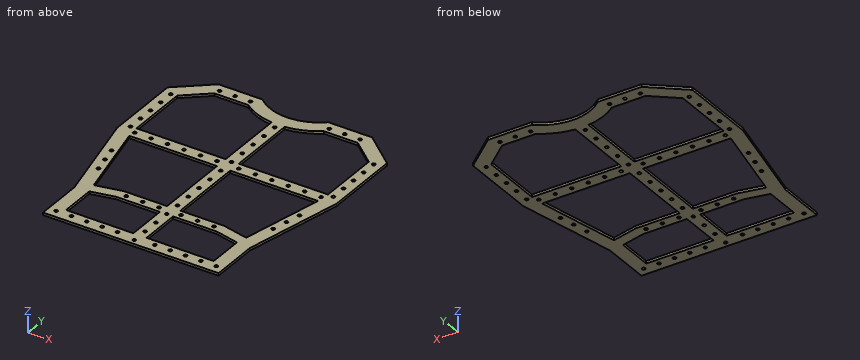
from build123d import *

# Parameters (mm, degrees)
BOSS_EXTRUDE1_DEPTH    = 2.286
SKETCH8_W              = 160
SKETCH8_H              = 1.5
CUT_EXTRUDE3_DEPTH     = 10
CUT_EXTRUDE4_DEPTH     = 3.286
BOSS_EXTRUDE2_DEPTH    = 2.286
F_3_0MM_DOWEL_HOLE4_D  = 3
F_3_0MM_DOWEL_HOLE5_D  = 3
F_3_0MM_DOWEL_HOLE6_D  = 3
F_3_0MM_DOWEL_HOLE7_D  = 3
F_3_0MM_DOWEL_HOLE8_D  = 3
F_3_0MM_DOWEL_HOLE9_D  = 3
F_3_0MM_DOWEL_HOLE10_D = 3


with BuildPart() as part:
    # Sketch1 → Boss-Extrude1 (new body)
    with BuildSketch(Plane.XY):
        with BuildLine():
            Line((-30, 6.458980338), (-70, 6.458980338))
            Line((-70, 6.458980338), (-100, -18.541019662))
            Line((-100, -18.541019662), (-100, -88.541019662))
            Line((-100, -88.541019662), (-80, -178.541019662))
            Line((-80, -178.541019662), (-80, -223.541019662))
            Line((-80, -223.541019662), (80, -223.541019662))
            Line((80, -223.541019662), (80, -178.541019662))
            Line((80, -178.541019662), (100, -88.541019662))
            Line((100, -88.541019662), (100, -18.541019662))
            Line((100, -18.541019662), (70, 6.458980338))
            Line((70, 6.458980338), (30, 6.458980338))
            ThreePointArc((30, 6.458980338), (0, -5), (-30, 6.458980338))
        make_face()
    extrude(amount=BOSS_EXTRUDE1_DEPTH)

    # Sketch8 → Cut-Extrude3 (cut)
    with BuildSketch(Plane.XY.offset(2.286)):
        with Locations((0, -222.791019662)):
            Rectangle(SKETCH8_W, SKETCH8_H)
    extrude(amount=-CUT_EXTRUDE3_DEPTH, mode=Mode.SUBTRACT)

    # Sketch15 → Cut-Extrude4 (cut, through all)
    with BuildSketch(Plane.XY.offset(2.286)):
        with BuildLine():
            Line((-87.3, -24.489381476), (-87.3, -81.146912359))
            Line((-87.3, -81.146912359), (-6, -81.146912359))
            Line((-6, -81.146912359), (-6, -17.387193693))
            ThreePointArc((-6, -17.387193693), (-21.008544759, -13.739473826), (-34.511709615, -6.241019662))
            Line((-34.511709615, -6.241019662), (-65.401965823, -6.241019662))
            Line((-65.401965823, -6.241019662), (-87.3, -24.489381476))
        make_face()
        with BuildLine():
            Line((6, -81.146912359), (87.3, -81.146912359))
            Line((87.3, -81.146912359), (87.3, -24.489381476))
            Line((87.3, -24.489381476), (65.401965823, -6.241019662))
            Line((65.401965823, -6.241019662), (34.511709615, -6.241019662))
            ThreePointArc((34.511709615, -6.241019662), (21.008544759, -13.739473826), (6, -17.387193693))
            Line((6, -17.387193693), (6, -81.146912359))
        make_face()
        Polygon((-67.3, -209.341019662), (-6, -209.341019662), (-6, -93.146912359), (-85.966666667, -93.146912359), (-67.3, -177.146912359), align=None)
        Polygon((6, -93.146912359), (6, -209.341019662), (67.3, -209.341019662), (67.3, -177.146912359), (85.966666667, -93.146912359), align=None)
    extrude(amount=-CUT_EXTRUDE4_DEPTH, mode=Mode.SUBTRACT)

    # Sketch16 → Boss-Extrude2 (add)
    with BuildSketch(Plane.XY.offset(2.286)):
        Polygon((-67.3, -177.146912359), (-46, -172.413579025), (-6, -172.413579025), (-6, -162.413579025), (-46, -162.413579025), (-69.417647059, -167.617500594), align=None)
    boss_extrude2 = extrude(amount=-BOSS_EXTRUDE2_DEPTH)

    # Mirror1: Boss-Extrude2 across plane
    add(boss_extrude2.mirror(Plane(origin=(0, 0, 0), x_dir=(0, 0, 1), z_dir=(1, 0, 0))))

    # Ø3.0mm Dowel Hole4 (through all)
    with Locations(Plane.XY.offset(2.286)):
        with Locations((-85, -87.146912359), (-70, -87.146912359), (-55, -87.146912359), (-40, -87.146912359), (-25, -87.146912359), (-10, -87.146912359), (10, -87.146912359), (25, -87.146912359), (40, -87.146912359), (55, -87.146912359), (70, -87.146912359), (85, -87.146912359)):
            Hole(F_3_0MM_DOWEL_HOLE4_D / 2)

    # Ø3.0mm Dowel Hole5 (through all)
    with Locations(Plane.XY.offset(2.286)):
        with Locations((0, -22.146912359), (0, -37.146912359), (0, -52.146912359), (0, -67.146912359), (0, -82.146912359), (0, -97.146912359), (0, -112.146912359), (0, -127.146912359), (0, -142.146912359), (0, -157.146912359), (0, -172.146912359), (0, -187.146912359), (0, -202.146912359), (0, -217.146912359)):
            Hole(F_3_0MM_DOWEL_HOLE5_D / 2)

    # Ø3.0mm Dowel Hole6 (through all)
    with Locations(Plane.XY.offset(2.286)):
        with Locations((-40, -167.413579025), (-25, -167.413579025), (-10, -167.413579025), (10, -167.413579025), (25, -167.413579025), (40, -167.413579025)):
            Hole(F_3_0MM_DOWEL_HOLE6_D / 2)

    # Ø3.0mm Dowel Hole7 (through all)
    with Locations(Plane(origin=(0, 0, 0), x_dir=(-1, 0, 0), z_dir=(0, 0, -1))):
        with Locations((92.507, -25.541019662), (92.507, -39.541019662), (92.507, -53.541019662), (92.507, -67.541019662), (92.507, -81.541019662)):
            f_3_0mm_dowel_hole7 = Hole(F_3_0MM_DOWEL_HOLE7_D / 2)

    # Mirror2: Ø3.0mm Dowel Hole7 across plane
    add(f_3_0mm_dowel_hole7.mirror(Plane(origin=(0, 0, 0), x_dir=(0, 0, 1), z_dir=(1, 0, 0))), mode=Mode.SUBTRACT)

    # Ø3.0mm Dowel Hole8 (through all)
    with Locations(Plane(origin=(0, 0, 0), x_dir=(-1, 0, 0), z_dir=(0, 0, -1))):
        with Locations((-73, -214.548019662), (-59, -214.548019662), (-45, -214.548019662), (-31, -214.548019662), (-17, -214.548019662), (17, -214.548019662), (31, -214.548019662), (45, -214.548019662), (59, -214.548019662), (73, -214.548019662)):
            Hole(F_3_0MM_DOWEL_HOLE8_D / 2)

    # Ø3.0mm Dowel Hole9 (through all)
    with Locations(Plane.XY.offset(2.286)):
        with Locations((-64, -1.034019662), (-50, -1.034019662), (-36, -1.034019662), (36, -1.034019662), (50, -1.034019662), (64, -1.034019662)):
            Hole(F_3_0MM_DOWEL_HOLE9_D / 2)

    # Ø3.0mm Dowel Hole10 (through all)
    with Locations(Plane.XY.offset(2.286)):
        with Locations((-85.721962662, -118.251164374), (-82.684936253, -131.917783217), (-79.647909843, -145.584402059)):
            f_3_0mm_dowel_hole10 = Hole(F_3_0MM_DOWEL_HOLE10_D / 2)

    # Mirror3: Ø3.0mm Dowel Hole10 across plane
    add(f_3_0mm_dowel_hole10.mirror(Plane(origin=(0, 0, 0), x_dir=(0, 0, 1), z_dir=(1, 0, 0))), mode=Mode.SUBTRACT)


solid = part.part
Input: part model. Units: mm. Frame: model coordinates. Round coordinates to 2 decimals unless told otherwise and drop trailing zeros. Order: outer loops, then holes, each group sorted by start corner. A loop starts at its lowest first (then second) coordinate and runs counter-clockwise, first axis right, second up.
1. Cut plane C-C, the plane y = -9. Output: boundary loops of the cut face in (x, z), then the cut area to 3 significant figures.
The answers:
outline: (-88.55, 0) - (-68.71, 0) - (-68.71, 2.29) - (-88.55, 2.29) - close; (-30.47, 0) - (30.47, 0) - (30.47, 2.29) - (-30.47, 2.29) - close; (68.71, 0) - (88.55, 0) - (88.55, 2.29) - (68.71, 2.29) - close
area: 230 mm2
2. Cut plane A-A, the plane y = -45.5. Output: boundary loops of the cut face in (x, z), then the cut area to 3 significant figures.
The answers:
outline: (-100, 0) - (-87.3, 0) - (-87.3, 2.29) - (-100, 2.29) - close; (-6, 0) - (6, 0) - (6, 2.29) - (-6, 2.29) - close; (87.3, 0) - (100, 0) - (100, 2.29) - (87.3, 2.29) - close
area: 85.5 mm2
3. Cut plane B-B, the plane z = 1.25. State how many separate pieces and enclosed holes the cut face has, then the cut area to 3 significant figures.
The answers:
separate pieces: 1
enclosed holes: 70
area: 14,500 mm2
4. Material intervals for line 1 (X direction, y = -202.5, z = 1.45); line 2 (X direction, y = -78.5, z = 1.65); line 3 (X direction, y = -205.5, z = 1.55), sorted ascending.
The answers:
line 1: x = -80 to -67.3, -6 to -1.46, 1.46 to 6, 67.3 to 80
line 2: x = -100 to -87.3, -6 to 6, 87.3 to 100
line 3: x = -80 to -67.3, -6 to 6, 67.3 to 80
